Build history of the part. All positions in model axes, mm. A direction names the side the tool comes from. Round coordinates to 2 decimals unless told otherwise and drop trailing zeros. Write each loop counter-clockwise with the first axis right and the second up, starting at its lowest first coordinate (ties: lowest second). Pieces come first, ordered by that corner, then holes.
from build123d import *

# Parameters (mm, degrees)
SKETCH1_W           = 32
SKETCH1_H           = 17
SKETCH1_R           = 4.25
BOSS_EXTRUDE1_DEPTH = 3
BOSS_EXTRUDE2_DEPTH = 24.2
SKETCH3_W           = 32
SKETCH3_H           = 17
SKETCH3_R           = 4.25
BOSS_EXTRUDE3_DEPTH = 3
BOSS_EXTRUDE4_DEPTH = 129.8
SKETCH5_W           = 32
SKETCH5_H           = 17
BOSS_EXTRUDE5_DEPTH = 18
SKETCH6_W           = 25
SKETCH6_H           = 3
CUT_EXTRUDE1_DEPTH  = 15
BOSS_EXTRUDE6_DEPTH = 17
SKETCH8_R           = 6
CUT_EXTRUDE2_DEPTH  = 46
SKETCH9_R           = 1.5875
SKETCH9_R_2         = 2.114349704
CUT_EXTRUDE3_DEPTH  = 46
SKETCH10_R          = 1.5875
SKETCH10_R_2        = 2.114349704
CUT_EXTRUDE4_DEPTH  = 4


with BuildPart() as part:
    # Sketch1 → Boss-Extrude1 (new body)
    with BuildSketch(Plane.XY):
        Rectangle(SKETCH1_W, SKETCH1_H)
        Circle(SKETCH1_R, mode=Mode.SUBTRACT)
    extrude(amount=BOSS_EXTRUDE1_DEPTH)

    # Sketch2 → Boss-Extrude2 (add)
    with BuildSketch(Plane.XY.offset(3)):
        with BuildLine():
            Line((-7.5, 1), (-7.5, 8.5))
            Line((-7.5, 8.5), (-16, 8.5))
            Line((-16, 8.5), (-16, -8.5))
            Line((-16, -8.5), (16, -8.5))
            Line((16, -8.5), (16, 8.5))
            Line((16, 8.5), (7.5, 8.5))
            Line((7.5, 8.5), (7.5, 1))
            ThreePointArc((7.5, 1), (0, -6.5), (-7.5, 1))
        make_face()
    extrude(amount=BOSS_EXTRUDE2_DEPTH)

    # Sketch3 → Boss-Extrude3 (add)
    with BuildSketch(Plane.XY.offset(27.2)):
        Rectangle(SKETCH3_W, SKETCH3_H)
        Circle(SKETCH3_R, mode=Mode.SUBTRACT)
    extrude(amount=BOSS_EXTRUDE3_DEPTH)

    # Sketch4 → Boss-Extrude4 (add)
    with BuildSketch(Plane.XY.offset(30.2)):
        with BuildLine():
            Line((16, -8.5), (-16, -8.5))
            Line((-16, -8.5), (-16, 8.5))
            Line((-16, 8.5), (-7.5, 8.5))
            Line((-7.5, 8.5), (-7.5, 1))
            ThreePointArc((-7.5, 1), (0, -6.5), (7.5, 1))
            Line((7.5, 1), (7.5, 8.5))
            Line((7.5, 8.5), (16, 8.5))
            Line((16, 8.5), (16, -8.5))
        make_face()
    extrude(amount=BOSS_EXTRUDE4_DEPTH)

    # Sketch5 → Boss-Extrude5 (add)
    with BuildSketch(Plane.XY.offset(160)):
        Rectangle(SKETCH5_W, SKETCH5_H)
    extrude(amount=BOSS_EXTRUDE5_DEPTH)

    # Sketch6 → Cut-Extrude1 (cut)
    with BuildSketch(Plane(origin=(0, 8.5, 0), x_dir=(1, 0, 0), z_dir=(0, 1, 0))):
        with Locations((0, -161.5)):
            Rectangle(SKETCH6_W, SKETCH6_H)
    extrude(amount=-CUT_EXTRUDE1_DEPTH, mode=Mode.SUBTRACT)

    # Sketch7 → Boss-Extrude6 (add)
    with BuildSketch(Plane(origin=(0, 8.5, 0), x_dir=(1, 0, 0), z_dir=(0, 1, 0))):
        with BuildLine():
            Line((-16, -178), (16, -178))
            Line((16, -178), (16, -192))
            ThreePointArc((16, -192), (13.071067812, -199.071067812), (6, -202))
            Line((6, -202), (-6, -202))
            ThreePointArc((-6, -202), (-13.071067812, -199.071067812), (-16, -192))
            Line((-16, -192), (-16, -178))
        make_face()
    extrude(amount=-BOSS_EXTRUDE6_DEPTH)

    # Sketch8 → Cut-Extrude2 (cut)
    with BuildSketch(Plane(origin=(0, 8.5, 0), x_dir=(1, 0, 0), z_dir=(0, 1, 0))):
        with Locations((0, -187)):
            Circle(SKETCH8_R)
    extrude(amount=-CUT_EXTRUDE2_DEPTH, mode=Mode.SUBTRACT)

    # Sketch9 → Cut-Extrude3 (cut)
    with BuildSketch(Plane(origin=(0, 8.5, 0), x_dir=(1, 0, 0), z_dir=(0, 1, 0))):
        with Locations((11.75, -130)):
            Circle(SKETCH9_R)
        with Locations((-11.75, -130)):
            Circle(SKETCH9_R)
        with Locations((11.75, -95)):
            Circle(SKETCH9_R)
        with Locations((-11.75, -95)):
            Circle(SKETCH9_R)
        with Locations((11.75, -60)):
            Circle(SKETCH9_R)
        with Locations((11.75, -25)):
            Circle(SKETCH9_R)
        with Locations((-11.75, -25)):
            Circle(SKETCH9_R)
        with Locations((-11.75, -60)):
            Circle(SKETCH9_R)
        with Locations((11.75, -168)):
            Circle(SKETCH9_R_2)
        with Locations((-11.75, -168)):
            Circle(SKETCH9_R_2)
    extrude(amount=-CUT_EXTRUDE3_DEPTH, mode=Mode.SUBTRACT)

    # Sketch10 → Cut-Extrude4 (cut)
    with BuildSketch(Plane.XZ.offset(8.5)):
        Polygon((-15.214, 25), (-13.482, 22), (-10.018, 22), (-8.286, 25), (-10.018, 28), (-13.482, 28), align=None)
        with Locations((-11.75, 25)):
            Circle(SKETCH10_R, mode=Mode.SUBTRACT)
        Polygon((13.482, 28), (10.018, 28), (8.286, 25), (10.018, 22), (13.482, 22), (15.214, 25), align=None)
        with Locations((11.75, 25)):
            Circle(SKETCH10_R, mode=Mode.SUBTRACT)
        Polygon((13.482, 171.283743046), (10.018, 171.283743046), (8.286, 168.283743046), (10.018, 165.283743046), (13.482, 165.283743046), (15.214, 168.283743046), align=None)
        with Locations((11.75, 168)):
            Circle(SKETCH10_R_2, mode=Mode.SUBTRACT)
        Polygon((-10.017949192, 57), (-8.285898385, 60), (-10.017949192, 63), (-13.482050808, 63), (-15.214101615, 60), (-13.482050808, 57), align=None)
        with Locations((-11.75, 60)):
            Circle(SKETCH10_R, mode=Mode.SUBTRACT)
        Polygon((13.482050808, 57), (15.214101615, 60), (13.482050808, 63), (10.017949192, 63), (8.285898385, 60), (10.017949192, 57), align=None)
        with Locations((11.75, 60)):
            Circle(SKETCH10_R, mode=Mode.SUBTRACT)
        Polygon((13.482050808, 92), (15.214101615, 95), (13.482050808, 98), (10.017949192, 98), (8.285898385, 95), (10.017949192, 92), align=None)
        with Locations((11.75, 95)):
            Circle(SKETCH10_R, mode=Mode.SUBTRACT)
        Polygon((-10.017949192, 92), (-8.285898385, 95), (-10.017949192, 98), (-13.482050808, 98), (-15.214101615, 95), (-13.482050808, 92), align=None)
        with Locations((-11.75, 95)):
            Circle(SKETCH10_R, mode=Mode.SUBTRACT)
        Polygon((-10.017949192, 127.2), (-8.285898385, 130.2), (-10.017949192, 133.2), (-13.482050808, 133.2), (-15.214101615, 130.2), (-13.482050808, 127.2), align=None)
        Polygon((-10.017949192, 165), (-8.285898385, 168), (-10.017949192, 171), (-13.482050808, 171), (-15.214101615, 168), (-13.482050808, 165), align=None)
        with Locations((-11.75, 168)):
            Circle(SKETCH10_R_2, mode=Mode.SUBTRACT)
        Polygon((10.04912113, 127.250391955), (13.280790983, 127.152191667), (14.981669853, 129.901799713), (13.45087887, 132.749608045), (10.219209017, 132.847808333), (8.518330147, 130.098200287), align=None)
    extrude(amount=-CUT_EXTRUDE4_DEPTH, mode=Mode.SUBTRACT)


solid = part.part
1) Mould opens along Z. For faces 4 (the flat face through (-4, 2, 0)), 5 (the cylindrical face through (2.285, 3.584, 1.479)), 6 (the cylindrical face through (-11.957, 2.091, 93.426)) say: released by +Z, released by -Z, zero draft, split by the parting line, or undercut.
Results:
face 4: released by -Z
face 5: zero draft
face 6: undercut
2) Wall check: L1, parallel to X at y = 3, z = 60; L2, parallel to X at y = -1.5, z = 168; L3, parallel to X at y = -0.75, z = 25. Give the ranges that are in metal, low to high.
Results:
L1: x = -16 to -13.34, -10.16 to -7.5, 7.5 to 10.16, 13.34 to 16
L2: x = -16 to -13.86, -9.64 to 9.64, 13.86 to 16
L3: x = -16 to -13.34, -10.16 to -7.29, 7.29 to 10.16, 13.34 to 16
3) Pin check, flat tips, straight feed: pin 1 Ø5 at (x, z) = (-11.75, 95) entering from +Y; pin 2 Ø1 at (x, y) = (12.5, -6) entering from +Z; pin 3 Ø3 at (x, z) = (12.5, 169) entering from -Y; pin 4 Ø8 at (x, z) = (-1, 64.5) entering from +Y. Stop position of each tip, or through.
Results:
pin 1: stops at y = 8.5
pin 2: stops at z = 200
pin 3: stops at y = -4.5
pin 4: stops at y = -4.59
4) Which spindle directions (+Z, -Z, +X, -X, +Y, -Y) get a long thin tool onto all of the face, cutting with end or side? Do faces 1 (the flat face through (-0.1, 4.4, 27.2)), 2 (the flat face through (12, -7, 22)), 3 (the cylindrical face through (11.543, 2.091, 58.426)). Say none if no direction does.
Results:
face 1: +Y
face 2: -Y
face 3: +Y, -Y
5) Slice it at A-A (z = 77.5). Write the cut outline in (x, y), plus the area to 3 significant figures.
Results:
outline: (-16, -8.5) - (16, -8.5) - (16, 8.5) - (7.5, 8.5) - (7.5, 1) arc R7.5 cw to (-7.5, 1) - (-7.5, 8.5) - (-16, 8.5) - close
area: 343 mm2
